Part print with two shaded views. Sizes in mm from the minimum x, y, z corner. Coordinates: 2 decimals unless noted, no trailing zeros. Loops run counter-clockwise (first coordinate to the right, second up) from the corner with the lowest first, then second, coordinate; pieces in that order, holes last.
(1) Slice it at C-C (x = 3.25). Give the cut face in (y, z).
(2) Wall check: L1, parallel to Z at x = 5, y = 95; L2, parallel to Z at x = 0.5, y = 8.5; L3, parallel to Y at x = 4, z = 57. Give the ranges that are in metal, low to high.
(3) Slice it at A-A (z = 90). Give the cut face in (x, y).
(4) Slice it at B-B (y = 105.5). Give the cut face in (x, z).
(5) Flat gauge pins, fed straight in: P1, Ø2, axis at x = 3, y = 52.5, coming from the +Z side; P2, Ø5, axis at x = 3, z = 88.5, coming from the -Y side; P3, Ø3, axis at x = 6.5, y = 98.5, coming from the -Z side. Where does each tip first touch, or does it go through?
(6) Slice it at D-D (z = 58). Give the cut face in (x, y).
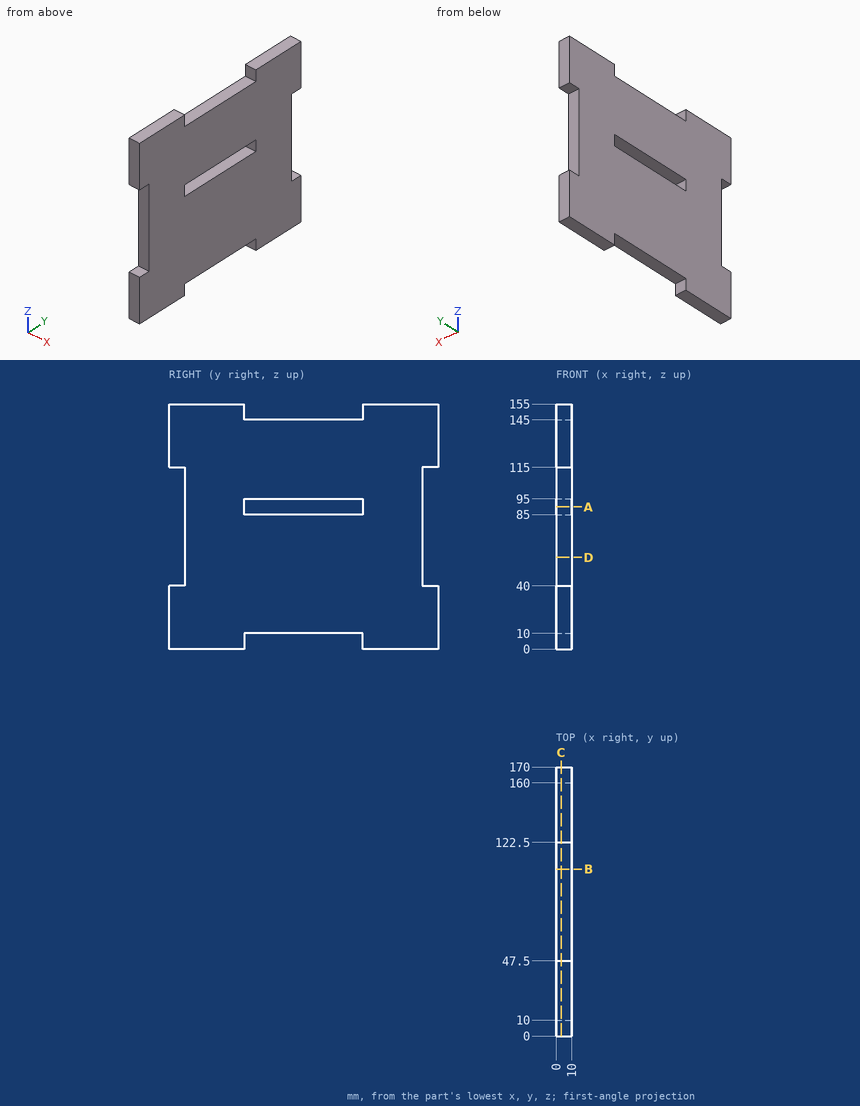
Response values:
1. outline: (0, 0) - (47.5, 0) - (47.5, 10) - (122.5, 10) - (122.5, 0) - (170, 0) - (170, 40) - (160, 40) - (160, 115) - (170, 115) - (170, 155) - (122.5, 155) - (122.5, 145) - (47.5, 145) - (47.5, 155) - (0, 155) - (0, 115) - (10, 115) - (10, 40) - (0, 40) - close; hole (47.5, 85) - (122.5, 85) - (122.5, 95) - (47.5, 95) - close
2. L1: z = 10 to 85, 95 to 145
2. L2: z = 0 to 40, 115 to 155
2. L3: y = 10 to 160
3. outline: (0, 10) - (10, 10) - (10, 47.5) - (0, 47.5) - close; (0, 122.5) - (10, 122.5) - (10, 160) - (0, 160) - close
4. outline: (0, 10) - (10, 10) - (10, 85) - (0, 85) - close; (0, 95) - (10, 95) - (10, 145) - (0, 145) - close
5. P1: stops at z = 145
5. P2: stops at y = 10
5. P3: stops at z = 10
6. outline: (0, 10) - (10, 10) - (10, 160) - (0, 160) - close
